Here's how the part is built. I have some questions about the finished solid (model axes, mm). Face numbers are marked on the shaded views. A direction names the side the tool comes from. Coordinates: 2 decimals unless noted, no trailing zeros. Write each loop counter-clockwise with the first axis right and the second up, starting at its lowest first coordinate (ties: lowest second). Pieces come first, ordered by that corner, then holes. Notation, with made-up numbers: (-14, 20.5) -> (30, 20.5) arc R25 cw to (30, 58.5) -> close; hole circle Ø3 at (57.5, 85). An arc over 180 degrees is marked (long way). Use a Markdown table: item, result. Add a question column.
Item 1: On a 3-axis mill with a long thin cutter (end or side, diameter ignored), from which of +Z, -Z, +X, -X, +Y, -Y can I reach the whole of each face in a straight line? I mean the marked faces 1 and 2. Say none if no direction works.
Item 2: Will these pins go through, and if not, where does the flat tip stop? pin 1 Ø1 at (x, z) = (0.5, 1) entering from +Y; pin 2 Ø1 at (x, z) = (-0.5, -3) entering from -Y; pin 3 Ø1.5 at (x, z) = (-0.5, -2.5) entering from -Y.
Item 3: Imagine slicing it at D-D, the plane z = 4.5. Write out the boundary of the cut face in (x, y), and give its area (3 significant figures).
Item 4: If I drill on line 1 along Y through (x, z) = (0.85, 0); line 2 along X through (y, z) = (3, 2.5); line 3 along Z through (x, y) = (-0.1, -1), over which ranges is the centre line in solid material (lowest first)? Write a range as from..to.
Item 5: Imagine slicing it at A-A, the plane y = 0. Write out the boundary of the cut face in (x, z), and give its area (3 significant figures).
Item 6: If we mould it in two halves opening along Y, with no side actions, what happens to the marked faces 3 and 4? For each: pulls with the +Y half, pulls with the -Y half, needs draft (parallel to the pull), parting line crosses it, or undercut.
Item 7: Imagine slicing it at C-C, the plane x = -1.1. Write out the boundary of the cut face in (y, z), and give its area (3 significant figures).
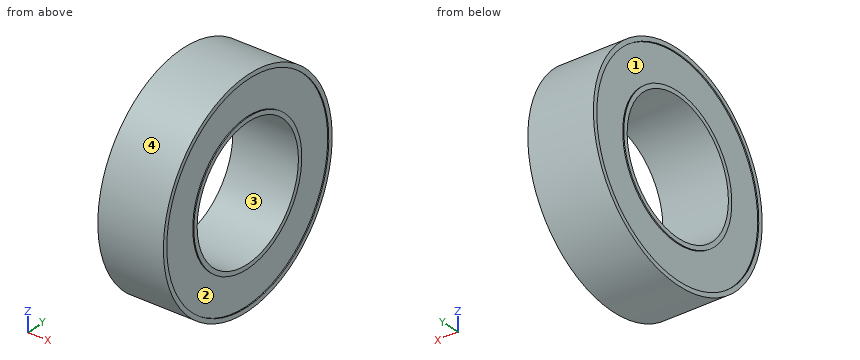
```python
from build123d import *

# Parameters (mm, degrees)
SKETCH1_R           = 5
SKETCH1_R_2         = 3
BOSS_EXTRUDE1_DEPTH = 1.5
SKETCH2_R           = 4.8
SKETCH2_R_2         = 3.2
CUT_EXTRUDE1_DEPTH  = 0.05


with BuildPart() as part:
    # Sketch1 → Boss-Extrude1 (new, symmetric)
    with BuildSketch(Plane(origin=(0, 0, 0), x_dir=(0, 0, -1), z_dir=(1, 0, 0))):
        Circle(SKETCH1_R)
        Circle(SKETCH1_R_2, mode=Mode.SUBTRACT)
    extrude(amount=BOSS_EXTRUDE1_DEPTH, both=True)

    # Sketch2 → Cut-Extrude1 (cut)
    with BuildSketch(Plane(origin=(1.5, 0, 0), x_dir=(0, 0, -1), z_dir=(1, 0, 0))):
        Circle(SKETCH2_R)
        Circle(SKETCH2_R_2, mode=Mode.SUBTRACT)
    cut_extrude1 = extrude(amount=-CUT_EXTRUDE1_DEPTH, mode=Mode.SUBTRACT)

    # Mirror1: Cut-Extrude1 across plane
    add(cut_extrude1.mirror(Plane(origin=(0, 0, 0), x_dir=(0, 0, 1), z_dir=(1, 0, 0))), mode=Mode.SUBTRACT)


solid = part.part
```
Ans:
| question | item | result |
|---|---|---|
| 1 | face 1 | -X |
| 1 | face 2 | +X |
| 2 | pin 1 | stops at y = 4.97 |
| 2 | pin 2 | stops at y = -4.33 |
| 2 | pin 3 | stops at y = -4.68 |
| 3 | outline | (-1.5, -2.18) -> (1.5, -2.18) -> (1.5, -1.67) -> (1.45, -1.67) -> (1.45, 1.67) -> (1.5, 1.67) -> (1.5, 2.18) -> (-1.5, 2.18) -> (-1.5, 1.67) -> (-1.45, 1.67) -> (-1.45, -1.67) -> (-1.5, -1.67) -> close |
| 3 | area | 12.7 mm^2 |
| 4 | line 1 | y = -5..-3, 3..5 |
| 4 | line 2 | x = -1.45..1.45 |
| 4 | line 3 | z = -4.9..-2.83, 2.83..4.9 |
| 5 | outline | (-1.5, -5) -> (1.5, -5) -> (1.5, -4.8) -> (1.45, -4.8) -> (1.45, -3.2) -> (1.5, -3.2) -> (1.5, -3) -> (-1.5, -3) -> (-1.5, -3.2) -> (-1.45, -3.2) -> (-1.45, -4.8) -> (-1.5, -4.8) -> close; (-1.5, 3) -> (1.5, 3) -> (1.5, 3.2) -> (1.45, 3.2) -> (1.45, 4.8) -> (1.5, 4.8) -> (1.5, 5) -> (-1.5, 5) -> (-1.5, 4.8) -> (-1.45, 4.8) -> (-1.45, 3.2) -> (-1.5, 3.2) -> close |
| 5 | area | 11.7 mm^2 |
| 6 | face 3 | undercut |
| 6 | face 4 | parting line crosses it |
| 7 | outline | circle Ø10 at (0, 0); hole circle Ø6 at (0, 0) |
| 7 | area | 50.3 mm^2 |
